from build123d import *

# Parameters (mm, degrees)
SKETCH1_R           = 50
BOSS_EXTRUDE1_DEPTH = 20
SKETCH2_R           = 25
SKETCH2_R_2         = 12.5
BOSS_EXTRUDE2_DEPTH = 40
FILLET1_R           = 2
FILLET2_R           = 2
SKETCH3_R           = 3.136270049
CUT_EXTRUDE1_DEPTH  = 25


with BuildPart() as part:
    # Sketch1 → Boss-Extrude1 (new body)
    with BuildSketch(Plane(origin=(0, 0, 0), x_dir=(1, 0, 0), z_dir=(0, 1, 0))):
        with Locations(Location((0, 0, 0), (0, 0, 270))):
            Circle(SKETCH1_R)
    extrude(amount=BOSS_EXTRUDE1_DEPTH)

    # Sketch2 → Boss-Extrude2 (add)
    with BuildSketch(Plane(origin=(0, 20, 0), x_dir=(1, 0, 0), z_dir=(0, 1, 0))):
        with Locations(Location((0, 0, 0), (0, 0, 270))):
            Circle(SKETCH2_R)
        with Locations(Location((0, 0, 0), (0, 0, 270))):
            Circle(SKETCH2_R_2, mode=Mode.SUBTRACT)
    extrude(amount=BOSS_EXTRUDE2_DEPTH)

    # Fillet1
    fillet1_edges = [part.edges().sort_by_distance(p)[0] for p in [
        (0, 0, -50),
    ]]
    fillet(fillet1_edges, radius=FILLET1_R)

    # Fillet2
    fillet2_edges = [part.edges().sort_by_distance(p)[0] for p in [
        (0, 20, -50),
        (0, 60, -25),
        (0, 20, -25),
    ]]
    fillet(fillet2_edges, radius=FILLET2_R)

    # Sketch3 → Cut-Extrude1 (cut, symmetric)
    with BuildSketch(Plane(origin=(0, 0, 0), x_dir=(0, 0, -1), z_dir=(1, 0, 0))):
        with Locations((0, 35)):
            Circle(SKETCH3_R)
    extrude(amount=CUT_EXTRUDE1_DEPTH, both=True, mode=Mode.SUBTRACT)


solid = part.part
Here's how the part is built. I have some questions about the finished solid (model axes, mm). A direction names the side the tool comes from. Round coordinates to 2 decimals unless told otherwise and drop trailing zeros. Order: outer loops, then holes, each group sorted by start corner. A loop starts at its lowest first (then second) coordinate and runs counter-clockwise, first axis right, second up. Notation, with made-up numbers: M 84.25,31.25 L 123.25,31.25 A22 ccw 123.25,68.25 Z; hole C 13.25,62 d1. An arc over 180 degrees is marked long. Return JSON: item names as keys, results as strings. Group by question number.
1. If we section it at B-B on x = 0: List the corners of the cut face in (y, z) for me.
2. If we section it at D-D on y = 47: List the corners of the cut face in (x, z) for me.
3. If we section it at C-C on y = 35: List the corners of the cut face in (x, z) for me.
4. I'm going to push flat-ended pins straight in: pin 1 Ø8 at (x, y) = (7, 37) entering from +Z; pin 2 Ø12 at (y, z) = (10, -37.5) entering from -X; pin 3 Ø10 at (x, y) = (-24, 33) entering from +Z; pin 4 Ø5 at (y, z) = (35, 0) entering from +X. Where does each tip first touch, or does it pass through?
5. If we section it at A-A on z = 0: List the corners of the cut face in (x, y) for me, then the cut area to 3 significant figures.
6. If we mould it in two halves opening along Y, with no side actions, what happens to faces 1 (the face through (-21, 20, 21)), 2 (the face through (15.02, 9.89, 47.69)), 3 (the face through (-18.46, 38.11, 0.41))? For each: pulls with the +Y half, pulls with the -Y half, needs draft (parallel to the pull), parting line crosses it, or undercut.
7. Please list where these lines run through material, in increasing order: probe 1 along X at (y, z) = (29.5, 0); probe 2 along Y at (x, z) = (18.5, 0); probe 3 along Y at (x, z) = (-36.5, -10).
8. On a 3-axis mill with a long thin cutter (end or side, diameter ignored), from which of +Z, -Z, +X, -X, +Y, -Y can I reach the whole of each face in a straight line? I mean faces 4 (the face through (1, 0, -1)), 5 (the face through (0, 20, 0)). Say none if no direction works.
Reply:
{
 "1": {"outline": "M 0,-48 A2 ccw 2,-50 L 18,-50 A2 ccw 20,-48 L 20,-27 A2 cw 22,-25 L 58,-25 A2 ccw 60,-23 L 60,-12.5 L 20,-12.5 L 20,12.5 L 60,12.5 L 60,23 A2 ccw 58,25 L 22,25 A2 cw 20,27 L 20,48 A2 ccw 18,50 L 2,50 A2 ccw 0,48 Z"},
 "2": {"outline": "C 0,0 d50; hole C 0,0 d25"},
 "3": {"outline": "M -24.8,-3.14 A25 ccw 24.8,-3.14 L 12.1,-3.14 A12.5 cw -12.1,-3.14 Z; M -24.8,3.14 L -12.1,3.14 A12.5 cw 12.1,3.14 L 24.8,3.14 A25 ccw Z"},
 "4": {"pin 1": "z = 24.82", "pin 2": "x = -38.83", "pin 3": "z = 16.25", "pin 4": "through"},
 "5": {"outline": "M -50,2 A2 ccw -48,0 L 48,0 A2 ccw 50,2 L 50,18 A2 ccw 48,20 L 27,20 A2 cw 25,22 L 25,31.86 L 12.5,31.86 L 12.5,20 L -12.5,20 L -12.5,31.86 L -25,31.86 L -25,22 A2 cw -27,20 L -48,20 A2 ccw -50,18 Z; M -25,38.14 L -12.5,38.14 L -12.5,60 L -23,60 A2 ccw -25,58 Z; M 12.5,38.14 L 25,38.14 L 25,58 A2 ccw 23,60 L 12.5,60 Z", "area": "2,840 mm^2"},
 "6": {"face 1": "pulls with the +Y half", "face 2": "needs draft", "face 3": "undercut"},
 "7": {"probe 1": "-25 to -12.5, 12.5 to 25", "probe 2": "0 to 31.86, 38.14 to 60", "probe 3": "0 to 20"},
 "8": {"face 4": "+Z, -Z, +X, -X, -Y", "face 5": "+Y"}
}
